Can you work these out from the model? Positions are in its coordinate system, mm. Face numbers are marked on the shaded views. Round coordinates to 2 decimals unless told otherwise and drop trailing zeros. Loops run counter-clockwise (first coordinate to the right, second up) from the corner with the lowest first, then second, coordinate; pieces in that order, holes last. Notation, with made-up numbers: (43, -17) -> (82, -17) arc R13 ccw to (82, 4) -> close; hole circle Ø4 at (59.5, 72.5). An arc over 180 degrees is marked (long way). Use a Markdown table: item, result.
from build123d import *

# Parameters (mm, degrees)
F0_W     = 81
F0_H     = 81
F1_DEPTH = 20
F2_W     = 71
F2_H     = 20.792734
F3_DEPTH = 81.001
F4_W     = 71
F4_H     = 29.603668
F5_DEPTH = 81.001
F6_R     = 3.75
F7_DEPTH = 20.001


with BuildPart() as f1:
    # F0 (on Top) → F1 (new body)
    with BuildSketch(Plane.XY):
        Rectangle(F0_W, F0_H)
        with BuildLine():
            ThreePointArc((-38.5, 18), (-30.052038, 30.052038), (-18, 38.5))
            Line((-18, 38.5), (18, 38.5))
            ThreePointArc((18, 38.5), (30.052038, 30.052038), (38.5, 18))
            Line((38.5, 18), (38.5, -18))
            ThreePointArc((38.5, -18), (30.052038, -30.052038), (18, -38.5))
            Line((18, -38.5), (-18, -38.5))
            ThreePointArc((-18, -38.5), (-30.052038, -30.052038), (-38.5, -18))
            Line((-38.5, -18), (-38.5, 18))
        make_face(mode=Mode.SUBTRACT)
    extrude(amount=F1_DEPTH)

    # F2 (on face) → F3 (cut, through all)
    with BuildSketch(Plane.XZ.offset(40.5)):
        with Locations((0, 6.603633)):
            Rectangle(F2_W, F2_H)
    extrude(amount=-F3_DEPTH, mode=Mode.SUBTRACT)

    # F4 (on face) → F5 (cut, through all)
    with BuildSketch(Plane(origin=(-40.5, 0, 0), x_dir=(0, -1, 0), z_dir=(-1, 0, 0))):
        with Locations((0, 2.198166)):
            Rectangle(F4_W, F4_H)
    extrude(amount=-F5_DEPTH, mode=Mode.SUBTRACT)

    # F6 (on face) → F7 (cut, through all)
    with BuildSketch(Plane.XY.offset(20)):
        with Locations((-36.25, 36.25)):
            Circle(F6_R)
        with Locations((36.25, 36.25)):
            Circle(F6_R)
        with Locations((-36.25, -36.25)):
            Circle(F6_R)
        with Locations((36.25, -36.25)):
            Circle(F6_R)
    extrude(amount=-F7_DEPTH, mode=Mode.SUBTRACT)


solid = f1.part
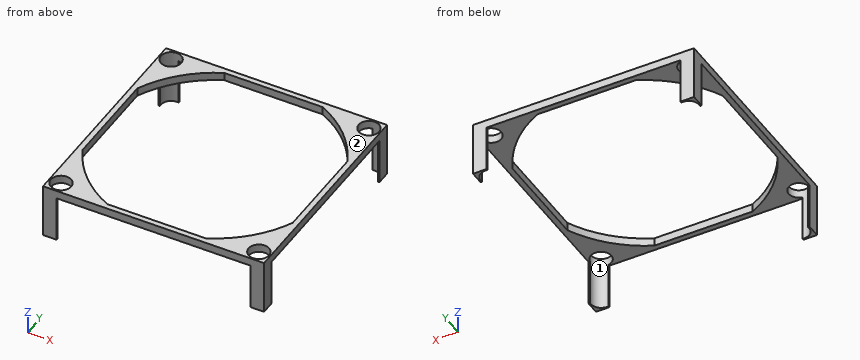
1. I want a section at B-B (x = -2.5). Please give me the cut outline in (y, z), plus the area to 3 significant figures.
Answer sheet:
| item | result |
|---|---|
| outline | (-40.5, 17) -> (-38.5, 17) -> (-38.5, 20) -> (-40.5, 20) -> close; (38.5, 17) -> (40.5, 17) -> (40.5, 20) -> (38.5, 20) -> close |
| area | 12.0 mm² |
2. If we mould it in two halves opening along Y, with no side actions, what happens to the marked faces 1 and 2? For each: +Y half, -Y half, draft (parallel to the pull), parting line (faces both ways), or undercut.
Answer sheet:
| item | result |
|---|---|
| face 1 | undercut |
| face 2 | draft |
3. Will this pin go through, and if not, where does the flat tip stop? pin 1 Ø12 at (x, z) = (-1.5, 7.5) entering from +Y.
Answer sheet:
| item | result |
|---|---|
| pin 1 | passes through |
4. I need wall thicknesses on line 1 (Y direction, x = 36.25, z = 14). Which ranges of the line are inside material? Lowest first, please.
Answer sheet:
| item | result |
|---|---|
| line 1 | y = -40.5 to -40, 40 to 40.5 |
5. I want a section at A-A (z = 9.75). Please give me the cut outline in (x, y), plus the area to 3 significant figures.
Answer sheet:
| item | result |
|---|---|
| outline | (-40.5, -40.5) -> (-35.5, -40.5) -> (-35.5, -39.92) arc R3.75 cw to (-39.92, -35.5) -> (-40.5, -35.5) -> close; (-40.5, 35.5) -> (-39.92, 35.5) arc R3.75 cw to (-35.5, 39.92) -> (-35.5, 40.5) -> (-40.5, 40.5) -> close; (35.5, -40.5) -> (40.5, -40.5) -> (40.5, -35.5) -> (39.92, -35.5) arc R3.75 cw to (35.5, -39.92) -> close; (35.5, 39.92) arc R3.75 cw to (39.92, 35.5) -> (40.5, 35.5) -> (40.5, 40.5) -> (35.5, 40.5) -> close |
| area | 31.2 mm² |
